```python
from build123d import *

# Parameters (mm, degrees)
SKETCH1_R               = 60
SKETCH1_R_2             = 54
BOSS_EXTRUDE1_DEPTH     = 3
SKETCH2_R               = 9
BOSS_EXTRUDE2_DEPTH     = 3
SKETCH3_R               = 8
BOSS_EXTRUDE3_DEPTH     = 5
BOSS_EXTRUDE4_DEPTH     = 3
CIRPATTERN9_COUNT       = 3
MIRROR2_COPY_1_DEPTH    = 3
MIRROR2_COPY_2_DEPTH    = 3
SKETCH5_R               = 1.5
CUT_EXTRUDE1_DEPTH      = 5
CUT_EXTRUDE2_DEPTH      = 86.229103011
CUT_EXTRUDE2_DEPTH_BACK = 86.229103011
SKETCH6_R               = 1.5
CUT_EXTRUDE3_DEPTH      = 86
CUT_EXTRUDE3_DEPTH_BACK = 86
SKETCH7_R               = 3.75


with BuildPart() as part:
    # Sketch1 → Boss-Extrude1 (new body)
    with BuildSketch(Plane(origin=(0, 0, 0), x_dir=(1, 0, 0), z_dir=(0, 1, 0))):
        with Locations(Location((0, 0, 0), (0, 0, 270))):
            Circle(SKETCH1_R)
        with Locations(Location((0, 0, 0), (0, 0, 270))):
            Circle(SKETCH1_R_2, mode=Mode.SUBTRACT)
    extrude(amount=BOSS_EXTRUDE1_DEPTH)



with BuildPart() as body_2:
    # Sketch2 → Boss-Extrude2 (new body)
    with BuildSketch(Plane(origin=(0, 0, 0), x_dir=(1, 0, 0), z_dir=(0, 1, 0))):
        with Locations(Location((0, 0, 0), (0, 0, 270))):
            Circle(SKETCH2_R)
    extrude(amount=BOSS_EXTRUDE2_DEPTH)

    # Sketch3 → Boss-Extrude3 (add)
    with BuildSketch(Plane(origin=(0, 3, 0), x_dir=(1, 0, 0), z_dir=(0, 1, 0))):
        with Locations(Location((0, 0, 0), (0, 0, 270))):
            Circle(SKETCH3_R)
    extrude(amount=BOSS_EXTRUDE3_DEPTH)


with BuildPart() as part_1:
    add(part.part)

    add(body_2.part)  # Boss-Extrude4 merges body 2
    # Sketch4 → Boss-Extrude4 (add)
    with BuildSketch(Plane(origin=(0, 0, 0), x_dir=(1, 0, 0), z_dir=(0, 1, 0))):
        with BuildLine():
            Line((9, 0), (54, 0))
            ThreePointArc((54, 0), (53.868998701, -3.759119436), (53.47663041, -7.5))
            ThreePointArc((53.47663041, -7.5), (52.338407888, -3.660460246), (48.694167528, -2))
            Line((48.694167528, -2), (16.899494937, -2))
            ThreePointArc((16.899494937, -2), (11.197705074, -3.13415652), (6.363961031, -6.363961031))
            ThreePointArc((6.363961031, -6.363961031), (8.314915793, -3.444150891), (9, 0))
        make_face()
    boss_extrude4 = extrude(amount=BOSS_EXTRUDE4_DEPTH)

    # CirPattern9: Boss-Extrude4 ×3 about axis
    cirpattern9_axis = Axis((0, 0, 0), (0, 1, 0))
    for i in range(1, CIRPATTERN9_COUNT):
        add(boss_extrude4.rotate(cirpattern9_axis, i * 360 / CIRPATTERN9_COUNT))

    # Mirror2: Boss-Extrude4 across plane
    add(boss_extrude4.mirror(Plane(origin=(-4.5, 54.446930959, -7.794228634), x_dir=(0.5000000000000041, 0, 0.8660254037844362), z_dir=(0.8660254037844364, 0, -0.5000000000000041))))

    # Mirror2 copy 1 sketch → Mirror2 copy 1 (add)
    with BuildSketch(Plane(origin=(0, 0, 0), x_dir=(-0.5000000000000082, 0, -0.8660254037844338), z_dir=(0, 1, 0))):
        with BuildLine():
            Line((9, 0), (54, 0))
            ThreePointArc((54, 0), (53.868998701, 3.759119436), (53.47663041, 7.5))
            ThreePointArc((53.47663041, 7.5), (52.338407888, 3.660460246), (48.694167528, 2))
            Line((48.694167528, 2), (16.899494937, 2))
            ThreePointArc((16.899494937, 2), (11.197705074, 3.13415652), (6.363961031, 6.363961031))
            ThreePointArc((6.363961031, 6.363961031), (8.314915793, 3.444150891), (9, 0))
        make_face()
    extrude(amount=MIRROR2_COPY_1_DEPTH)

    # Mirror2 copy 2 sketch → Mirror2 copy 2 (add)
    with BuildSketch(Plane(origin=(0, 0, 0), x_dir=(1, 0, 0), z_dir=(0, 1, 0))):
        with BuildLine():
            Line((9, 0), (54, 0))
            ThreePointArc((54, 0), (53.868998701, 3.759119436), (53.47663041, 7.5))
            ThreePointArc((53.47663041, 7.5), (52.338407888, 3.660460246), (48.694167528, 2))
            Line((48.694167528, 2), (16.899494937, 2))
            ThreePointArc((16.899494937, 2), (11.197705074, 3.13415652), (6.363961031, 6.363961031))
            ThreePointArc((6.363961031, 6.363961031), (8.314915793, 3.444150891), (9, 0))
        make_face()
    extrude(amount=MIRROR2_COPY_2_DEPTH)

    # Sketch5 → Cut-Extrude1 (cut)
    with BuildSketch(Plane(origin=(0, 8, 0), x_dir=(1, 0, 0), z_dir=(0, 1, 0))):
        with Locations(Location((5.5, 0, 0), (0, 0, 270))):
            Circle(SKETCH5_R)
    extrude(amount=-CUT_EXTRUDE1_DEPTH, mode=Mode.SUBTRACT)

    # Sketch6 → Cut-Extrude2 (cut, two sides: drawn at the far end of the back side and taken through both)
    with BuildSketch(Plane(origin=(0, 8, 0), x_dir=(1, 0, 0), z_dir=(0, 1, 0)).offset(-CUT_EXTRUDE2_DEPTH_BACK)):
        with Locations(Location((0, 0, 0), (0, 0, 270))):
            Circle(SKETCH6_R)
    extrude(amount=CUT_EXTRUDE2_DEPTH + CUT_EXTRUDE2_DEPTH_BACK, mode=Mode.SUBTRACT)

    # Sketch7 → Cut-Extrude3 (cut, two sides: drawn at the far end of the back side and taken through both)
    with BuildSketch(Plane(origin=(0, 3, 0), x_dir=(1, 0, 0), z_dir=(0, 1, 0)).offset(-CUT_EXTRUDE3_DEPTH_BACK)):
        with Locations(Location((55.25, 0, 0), (0, 0, 270))):
            Circle(SKETCH7_R)
    extrude(amount=CUT_EXTRUDE3_DEPTH + CUT_EXTRUDE3_DEPTH_BACK, mode=Mode.SUBTRACT)


solid = part_1.part
```
Source: CAD feature listing. Evaluate the final solid. Frame: model axes, mm. A direction names the side the tool comes from. Round coordinates to 2 decimals unless told otherwise and drop trailing zeros. Loops run counter-clockwise (first coordinate to the right, second up) from the corner with the lowest first, then second, coordinate; pieces in that order, holes last.
1. Contact query for flat-ended pins moving along their axis: pin 1 (1 mm diameter, centred on y = 1.5, z = 30, fed in from -X); pin 2 (0.9 mm diameter, centred on x = 6, z = -0.5, fed in from +Y); pin 3 (1 mm diameter, centred on x = -29.5, y = 2, fed in from +Z); pin 4 (3.5 mm diameter, centred on x = 5.5, z = 0, fed in from +Y). Output: stop coordinate, or through.
2. Mould query, pull axis Z, two halves, no side actions, for faces 1 (the cylindrical face through (2.64, 1.48, -59.94)), 2 (the cylindrical face through (-8.324, 1.479, -8.212)), 3 (the flat face through (0, 3, 9)). Classes: released by +Z, released by -Z, zero draft, split by the parting line, or undercut.
3. Section query A-A on z = 0. Output: boundary loops of the cut face in (x, y), and give its area (4 significant figures).
4. Access query for faces 4 (the cylindrical face through (-2.949, 1.479, -11.315)), 5 (the cylindrical face through (-7.81, 5.46, -1.73)). Directions: +Z, -Z, +X, -X, +Y, -Y. A direction counts if a zero-diameter tool reaches every point of the face in a straight line with its end or side. Return the directions, or none.
5. Section query B-B on x = 14. Output: boundary loops of the cut face in (y, z).
6. Ray query, L1, parallel to X at y = 5.45, z = 0; L2, parallel to Z at x = -22.5, y = 2; L3, parallel to Z at x = 42, y = 1.25. Return the intervals inside material, ascending.
7. Section query C-C on z = -52. Output: boundary loops of the cut face in (x, y), and give its area (3 significant figures).
8. Section query D-D on x = 0. Output: boundary loops of the cut face in (y, z).
Answers below:
1. pin 1: stops at x = -52.25
1. pin 2: stops at y = 3
1. pin 3: stops at z = 52.53
1. pin 4: stops at y = 8
2. face 1: split by the parting line
2. face 2: undercut
2. face 3: zero draft
3. outline: (-60, 0) - (-54, 0) - (-54, 3) - (-60, 3) - close; (-9, 0) - (-1.5, 0) - (-1.5, 8) - (-8, 8) - (-8, 3) - (-9, 3) - close; (1.5, 0) - (51.5, 0) - (51.5, 3) - (8, 3) - (8, 8) - (7, 8) - (7, 3) - (4, 3) - (4, 8) - (1.5, 8) - close; (59, 0) - (60, 0) - (60, 3) - (59, 3) - close
3. area: 243.5 mm2
4. face 4: +Y, -Y
4. face 5: +Y
5. outline: (0, -58.34) - (3, -58.34) - (3, -52.15) - (0, -52.15) - close; (0, -2.28) - (3, -2.28) - (3, 2.28) - (0, 2.28) - close; (0, 52.15) - (3, 52.15) - (3, 58.34) - (0, 58.34) - close
6. L1: x = -8 to -1.5, 1.5 to 4, 7 to 8
6. L2: z = -55.62 to -48.19, -42.97 to -34.97, 34.97 to 42.97, 48.19 to 55.62
6. L3: z = -42.85 to -33.94, -2 to 2, 33.94 to 42.85
7. outline: (-29.93, 0) - (-14.56, 0) - (-14.56, 3) - (-29.93, 3) - close; (14.56, 0) - (29.93, 0) - (29.93, 3) - (14.56, 3) - close
7. area: 92.2 mm2
8. outline: (0, -60) - (3, -60) - (3, -54) - (0, -54) - close; (0, -9.53) - (3, -9.53) - (3, -8) - (8, -8) - (8, -1.5) - (0, -1.5) - close; (0, 1.5) - (8, 1.5) - (8, 8) - (3, 8) - (3, 9.53) - (0, 9.53) - close; (0, 54) - (3, 54) - (3, 60) - (0, 60) - close
